Autodesk Inventor part; units mm, degrees
ref_plane "YZ Plane" through (0, 0, 0) normal (1, 0, 0) x (0, 1, 0)
ref_plane "XZ Plane" through (0, 0, 0) normal (0, 1, 0) x (-1, 0, 0)
ref_plane "XY Plane" through (0, 0, 0) normal (0, 0, 1) x (1, 0, 0)
sketch "Sketch1" plane through (0, 0, 0) normal (0, 1, 0) x (-1, 0, 0)
  line L0 (0, 0) -> (7.7978, 0)
  line L1 (7.7978, 0) -> (7.7978, -7.7978)
  line L2 (7.7978, -7.7978) -> (0, -7.7978)
  line L3 (0, -7.7978) -> (0, 0)
  dimension "d0" = 7.7978
  dimension "d8" = 7.7978
extrude "Extrusion1" add sketch "Sketch1" along normal blind 9.6088
sketch "Sketch2" plane through (0, 9.6088, 0) normal (0, 1, 0) x (1, 0, 0)
  line L0 (0, 0) -> (-3.8989, 0) construction
  line L1 (-3.8989, 0) -> (-3.8989, 3.8989) construction
  line L2 (-3.8989, 3.8989) -> (0, 3.8989) construction
  line L3 (0, 3.8989) -> (0, 0) construction
  circle A0 centre (-3.8989, 3.8989) radius 2.4498
  dimension "d11" = 3.8989
  dimension "d12" = 3.8989
  dimension "d13" = 4.8997
extrude "Extrusion2" add sketch "Sketch2" along normal blind 1.9837
shell "Shell1" thickness 1.4732 removed faces 1 at (-2.5993, 0, -2.5993)
sketch "Sketch3" plane through (-7.7978, 0, 0) normal (0, 0, 1) x (1, 0, 0)
  line L0 (0, 0) -> (0, 9.6088) construction
  line L1 (0, 9.6088) -> (3.8989, 9.6088) construction
  line L2 (3.8989, 9.6088) -> (3.8989, 5.7099) construction
  line L3 (3.8989, 5.7099) -> (0, 5.7099) construction
  line L4 (0, 5.7099) -> (0, 9.6088) construction
  circle A0 centre (3.8989, 5.7099) radius 2.4498
  point P0 (7.7978, 0)
  dimension "d17" = 3.8989
  dimension "d18" = 3.8989
  dimension "d19" = 4.8997
extrude "Extrusion3" add sketch "Sketch3" along normal blind 1.9837
sketch "Sketch4" plane through (-3.8989, 5.7099, 1.9837) normal (0, 0, 1) x (1, 0, 0)
  circle A0 centre (0, 0) radius 2.4498 construction
  circle A1 centre (0, 0) radius 1.618
  point P0 (3.8989, -5.7099)
  dimension "d22" = 3.236
extrude "Extrusion4" cut sketch "Sketch4" against normal up to surface (3.4569 mm away)
equation "\"d0\" = d1"
equation "\"d8\" = d1"
equation "\"d9\" = d3"
equation "\"d11\" = 0.5 * d1"
equation "\"d12\" = 0.5 * d1"
equation "\"d13\" = d4"
equation "\"d14\" = d5"
equation "\"d16\" = d6"
equation "\"d17\" = 0.5 * d1"
equation "\"d18\" = 0.5 * d1"
equation "\"d19\" = d4"
equation "\"d20\" = d5"
equation "\"d22\" = d2"
equation "\"d23\" = d5"
equation "\"d1\" = 7.7978"
equation "\"d2\" = 3.23596"
equation "\"d3\" = 9.60882"
equation "\"d4\" = 4.89966"
equation "\"d5\" = 1.98374"
equation "\"d6\" = 1.4732"
equation "\"d7\" = 1.23952"
properties part number "1x1 tall gray with a stick out" material "ABS Plastic"
Input: part model. Units: mm. Frame: model coordinates. A direction names the side the tool comes from. Give positions to 0.01 mm unless a question says otherwise; leave off trailing zeros. Loops run counter-clockwise (first coordinate to the right, second up) from the corner with the lowest first, then second, coordinate; pieces in that order, holes last. Notation, with made-up numbers: (83, -1) -> (104, -1) arc R14 cw to (104, 4) -> close; hole circle Ø11 at (23, -39). An arc over 180 degrees is marked (long way). Use a Markdown table: item, result.
Q1. First-contact query: P1, Ø0.6, axis at x = -3.5, z = -4, coming from the -Y side; P2, Ø1.5, axis at x = -5, z = -4.5, coming from the -Y side. Flat tips, straight axial feed; report the tip coordinate or a pass-through.
Entries:
| item | result |
|---|---|
| P1 | stops at y = 10.12 |
| P2 | stops at y = 8.14 |
Q2. Pull-direction query (X, two-part tool) for faces 1 (the flat face through (-1, 0, -4)), 2 (the flat face through (-7.798, 5, -4)), 3 (the cylindrical face through (-4.11, 7.314, 0.279)); classes: pulls with the +X half, pulls with the -X half, needs draft (parallel to the pull), parting line crosses it, or undercut.
Entries:
| item | result |
|---|---|
| face 1 | needs draft |
| face 2 | pulls with the -X half |
| face 3 | undercut |
Q3. Section query B-B, the plane x = -4. Return the cut outline in (y, z), plus the area to 3 significant figures.
Entries:
| item | result |
|---|---|
| outline | (0, -7.8) -> (9.61, -7.8) -> (9.61, -6.35) -> (11.59, -6.35) -> (11.59, -1.45) -> (9.61, -1.45) -> (9.61, 0) -> (8.16, 0) -> (8.16, 1.98) -> (7.32, 1.98) -> (7.32, -1.47) -> (8.14, -1.47) -> (8.14, -2.93) -> (10.12, -2.93) -> (10.12, -4.87) -> (8.14, -4.87) -> (8.14, -6.32) -> (0, -6.32) -> close; (0, -1.47) -> (4.1, -1.47) -> (4.1, 1.98) -> (3.26, 1.98) -> (3.26, 0) -> (0, 0) -> close |
| area | 39.9 mm² |
Q4. Section query C-C, the plane z = -3.25. Return the cut outline in (x, y), plus the area to 3 significant figures.
Entries:
| item | result |
|---|---|
| outline | (-7.8, 0) -> (-6.32, 0) -> (-6.32, 8.14) -> (-4.63, 8.14) -> (-4.63, 10.12) -> (-3.17, 10.12) -> (-3.17, 8.14) -> (-1.47, 8.14) -> (-1.47, 0) -> (0, 0) -> (0, 9.61) -> (-1.54, 9.61) -> (-1.54, 11.59) -> (-6.26, 11.59) -> (-6.26, 9.61) -> (-7.8, 9.61) -> close |
| area | 41.9 mm² |
Q5. Section query A-A, the plane y = 3. Return the cut outline in (x, z), plus the area to 3 significant figures.
Entries:
| item | result |
|---|---|
| outline | (-7.8, -7.8) -> (0, -7.8) -> (0, 0) -> (-7.8, 0) -> close; hole (-6.32, -6.32) -> (-1.47, -6.32) -> (-1.47, -1.47) -> (-6.32, -1.47) -> close |
| area | 37.3 mm² |
Q6. Ray query, probe 1 along X at (y, z) = (7, -5.25); probe 2 along Z at (x, y) = (-6.5, 7). Return the intervals inside material, ascending. Write a range as from..to.
Entries:
| item | result |
|---|---|
| probe 1 | x = -7.8..-6.32, -1.47..0 |
| probe 2 | z = -7.8..0 |
Q7. Section query D-D, the plane y = 6.5. Return the cut outline in (x, z), plus the area to 3 significant figures.
Entries:
| item | result |
|---|---|
| outline | (-7.8, -7.8) -> (0, -7.8) -> (0, 0) -> (-1.58, 0) -> (-1.58, 1.98) -> (-2.49, 1.98) -> (-2.49, -1.47) -> (-1.47, -1.47) -> (-1.47, -6.32) -> (-6.32, -6.32) -> (-6.32, -1.47) -> (-5.31, -1.47) -> (-5.31, 1.98) -> (-6.22, 1.98) -> (-6.22, 0) -> (-7.8, 0) -> close |
| area | 36.7 mm² |
Q8. Access query for faces 4 (the flat face through (0, 5, -4)), 5 (the cylindrical face through (-4.43, 8.1, 0.98)), 6 (the flat face through (-4, 3, -1.473)), 7 (the flat face through (-2, 9.609, -2)), 8 (the flat face through (-3, 4, 1.984)). Directions: +Z, -Z, +X, -X, +Y, -Y. A direction counts if a zero-diameter tool reaches every point of the face in a straight line with its end or side. Return the directions, or none.
Entries:
| item | result |
|---|---|
| face 4 | +Z, -Z, +X, +Y, -Y |
| face 5 | +Z |
| face 6 | -Y |
| face 7 | +Y |
| face 8 | +Z, +X, -X, +Y, -Y |
